Source: CAD feature listing. Evaluate the final solid. Frame: model axes, mm. A direction names the side the tool comes from. Coordinates: 2 decimals unless noted, no trailing zeros. Order: outer loops, then holes, each group sorted by start corner. A loop starts at its lowest first (then second) coordinate and runs counter-clockwise, first axis right, second up. Notation, with made-up numbers: (2, 50) - (37, 50) arc R21 ccw to (37, 61) - close; hole circle Ø4 at (-21.5, -9.75). An arc over 180 degrees is marked (long way). One line per question, with ' | ' between items. Start each with the question number.
(1) Access query for faces 5 (the flat face through (-24, 4, 12.7)), 6 (the cylindrical face through (-7.79, 17.92, 8.8)). Directions: +Z, -Z, +X, -X, +Y, -Y. A direction counts if a zero-diameter tool reaches every point of the face in a straight line with its end or side. Return the directions, or none.
(2) Section B-B (y = 15). Return the cut outline in (x, z).
(3) Contact query for flat-ended pins moving along their axis: P1, Ø2.5, axis at x = -24, y = 3, coming from the +Z side; P2, Ø12, axis at x = -31, y = 12, coming from the +Z side. Output: stop coordinate, or through.
(4) Section C-C (x = -24). Return the cut outline in (y, z).
(5) Section D-D (z = 3.25). Return the cut outline in (x, y) (1 decimal), then the cut area to 3 significant figures.
(6) Draft query along Y for faces 1 (the cylindrical face through (-31.368, 19.551, 1.288)), 2 (the cylindrical face through (-25.09, 4.48, 10.77)), 3 (the flat face through (-19, -13.525, 1)), 4 (the flat face through (-19, 6, 0)). Return one class per face: +Y half, -Y half, draft (parallel to the pull), parting line (faces both ways), or undercut.
(7) Line query: line 1 along Z through (x, y) = (-28, 19); line 2 along X through (y, z) = (20, 1.75); line 3 along Y through (x, z) = (-9, 12). Output: solid intervals per line, ascending.
(8) Section A-A (x = -29.5). Return the cut outline in (y, z), then the cut area to 3 significant figures.
from build123d import *

# Parameters (mm, degrees)
SKETCH1_W           = 38.1
SKETCH1_H           = 38.1
BOSS_EXTRUDE1_DEPTH = 2.54
SKETCH2_R           = 1.5875
SKETCH2_R_2         = 1.27
BOSS_EXTRUDE2_DEPTH = 12.7
SKETCH5_R           = 1.27
CUT_EXTRUDE1_DEPTH  = 48.83102763
SKETCH6_R           = 2.54
BOSS_EXTRUDE3_DEPTH = 6.35
CUT_EXTRUDE2_START  = -2.54
SKETCH7_R           = 1.5875
CUT_EXTRUDE2_DEPTH  = 2.54


with BuildPart() as part:
    # Sketch1 → Boss-Extrude1 (new body)
    with BuildSketch(Plane.XY):
        with Locations((-19.05, 5.525182688)):
            Rectangle(SKETCH1_W, SKETCH1_H)
    extrude(amount=BOSS_EXTRUDE1_DEPTH)

    # Sketch2 → Boss-Extrude2 (add)
    with BuildSketch(Plane.XY.offset(2.54)):
        with Locations(Location((-8.001, 19.495182688, 0), (0, 0, 180))):
            Circle(SKETCH2_R)
        with Locations(Location((-23.626645651, 3.869537037, 0), (0, 0, 180))):
            Circle(SKETCH2_R)
        with Locations(Location((-30.099, 19.495182688, 0), (0, 0, 180))):
            Circle(SKETCH2_R_2)
    extrude(amount=BOSS_EXTRUDE2_DEPTH)

    # Sketch5 → Cut-Extrude1 (cut, through all)
    with BuildSketch(Plane.XY.offset(15.24)):
        with Locations((-30.099, 19.495182688)):
            Circle(SKETCH5_R)
    extrude(amount=-CUT_EXTRUDE1_DEPTH, mode=Mode.SUBTRACT)

    # Sketch6 → Boss-Extrude3 (add)
    with BuildSketch(Plane.XY.offset(2.54)):
        with Locations((-23.626645651, 3.869537037)):
            Circle(SKETCH6_R)
    extrude(amount=BOSS_EXTRUDE3_DEPTH)

    # Sketch7 → Cut-Extrude2 (cut)
    with BuildSketch(Plane.XY.offset(15.24).offset(CUT_EXTRUDE2_START)):
        with Locations(Location((-23.626645651, 3.869537037, 0), (0, 0, 180))):
            Circle(SKETCH7_R)
    extrude(amount=CUT_EXTRUDE2_DEPTH, mode=Mode.SUBTRACT)


solid = part.part
Response values:
1) face 5: +Z, +X, -X, +Y, -Y | face 6: +Z
2) outline: (-38.1, 0) - (0, 0) - (0, 2.54) - (-38.1, 2.54) - close
3) P1: stops at z = 12.7 | P2: stops at z = 2.54
4) outline: (-13.52, 0) - (24.58, 0) - (24.58, 2.54) - (6.38, 2.54) - (6.38, 8.89) - (5.41, 8.89) - (5.41, 12.7) - (2.33, 12.7) - (2.33, 8.89) - (1.36, 8.89) - (1.36, 2.54) - (-13.52, 2.54) - close
5) outline: circle Ø5.1 at (-23.6, 3.9); circle Ø3.2 at (-8, 19.5) | area: 28.2 mm²
6) face 1: undercut | face 2: parting line | face 3: -Y half | face 4: draft
7) line 1: z = 0 to 2.54 | line 2: x = -38.1 to -31.26, -28.93 to 0 | line 3: y = 18.26 to 20.73
8) outline: (-13.52, 0) - (18.38, 0) - (18.38, 2.54) - (-13.52, 2.54) - close; (20.62, 0) - (24.58, 0) - (24.58, 2.54) - (20.62, 2.54) - close | area: 91.1 mm²
